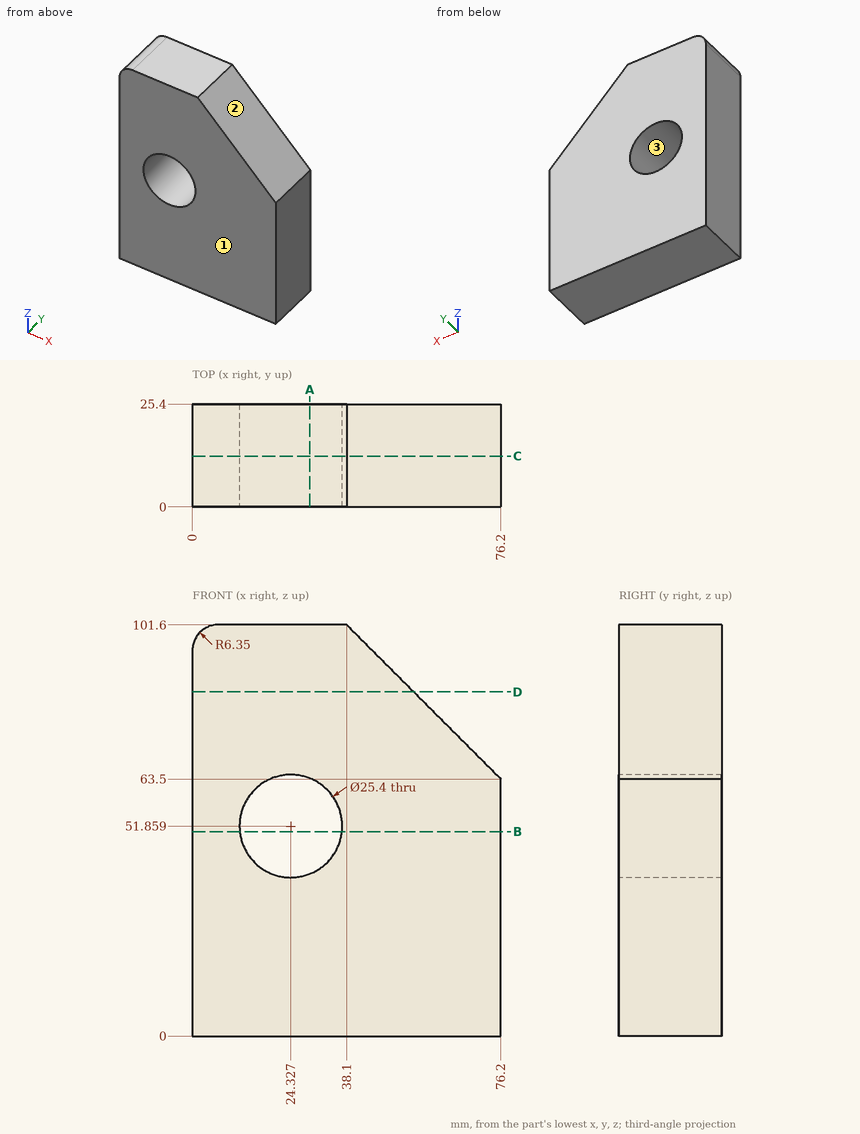
Could you check a few things on this drawing? It's one solid part, dimensions in mm from its lowest x, y, z. Give positions to 0.01 mm unless a question says otherwise; leave off trailing zeros. Loops run counter-clockwise (first coordinate to the right, second up) from the corner with the lowest first, then second, coordinate; pieces in that order, holes last. Notation, with made-up numbers: M 21.25,82 L 61.25,82 A13 ccw 61.25,89 Z; hole C -2,-28.5 d3. An arc over 180 degrees is marked long. Return JSON: item names as keys, results as strings.
Item 1: Please list where these lines run through material, in increasing order: line 1 (Z direction, x = 28, y = 20.5); line 2 (Z direction, x = 16.5, y = 8); line 3 (X direction, y = 13.5, z = 62.5) (1 decimal).
A:
{"line 1": "z = 0 to 39.7, 64.02 to 101.6", "line 2": "z = 0 to 41.86, 61.86 to 101.6", "line 3": "x = 0 to 17.4, 31.3 to 76.2"}
Item 2: Thinking about a two-plate mould opening in X: for the marked faces 1, 2 and 3, which applies, released by +X, released by -X, zero draft, split by the parting line, or undercut?
A:
{"face 1": "zero draft", "face 2": "released by +X", "face 3": "undercut"}
Item 3: Imagine slicing it at A-A on x = 29. List the corners of the cut face in (y, z) for me, then the cut area to 3 significant figures.
A:
{"outline": "M 0,0 L 25.4,0 L 25.4,40.05 L 0,40.05 Z; M 0,63.67 L 25.4,63.67 L 25.4,101.6 L 0,101.6 Z", "area": "1,980 mm^2"}
Item 4: Imagine slicing it at B-B on z = 50.5. List the corners of the cut face in (x, y) for me, then the cut area to 3 significant figures.
A:
{"outline": "M 0,0 L 11.7,0 L 11.7,25.4 L 0,25.4 Z; M 36.95,0 L 76.2,0 L 76.2,25.4 L 36.95,25.4 Z", "area": "1,290 mm^2"}
Item 5: Imagine slicing it at D-D on z = 85. List the corners of the cut face in (x, y) for me.
A:
{"outline": "M 0,0 L 54.7,0 L 54.7,25.4 L 0,25.4 Z"}
Item 6: Imagine slicing it at C-C on y = 12.5. List the corners of the cut face in (x, z) for me.
A:
{"outline": "M 0,0 L 76.2,0 L 76.2,63.5 L 38.1,101.6 L 6.35,101.6 A6.35 ccw 0,95.25 Z; hole C 24.33,51.86 d25.4"}
Item 7: I'm going to push flat-ended pins straight in: pin 1 Ø12 at (y, z) = (15, 76.5) entering from +X; pin 2 Ø6 at (x, y) = (62.5, 11.5) entering from -Z; pin 3 Ø5 at (x, y) = (55, 10.5) entering from +Z; pin 4 Ø20.5 at (x, z) = (24.33, 51.86) entering from -Y. Where does each tip first touch, or does it pass through?
A:
{"pin 1": "stops at x = 69.2", "pin 2": "stops at z = 0", "pin 3": "stops at z = 87.2", "pin 4": "passes through"}
